Read the model definition and answer for the solid it produces. Units are mm, in the model's axes. A direction names the side the tool comes from. Give positions to 0.01 mm unless a question says otherwise; leave off trailing zeros. Order: outer loops, then holes, each group sorted by start corner. A loop starts at its lowest first (then second) coordinate and runs counter-clockwise, first axis right, second up. Notation, with made-up numbers: (30.5, 88.5) - (79.5, 88.5) arc R25 ccw to (79.5, 105.5) - close; hole circle Ø4 at (28.5, 66). An arc over 180 degrees is marked (long way). Answer as CSV lines item,"result". Start each with the question number.
from build123d import *

# Parameters (mm, degrees)
F0_W     = 6
F0_H     = 6
F0_W_2   = 1
F0_H_2   = 5
F1_DEPTH = 1
F2_DEPTH = 6
F3_R     = 2.49999
F4_R     = 1
F5_DEPTH = 25


# Not quite as in the source:
# - a fillet or chamfer is up to 0.001 mm smaller than in the source, because OpenCascade refuses the exact size


with BuildPart() as f1:
    # F0 (on Top) → F1 (new body)
    with BuildSketch(Plane.XY):
        Rectangle(F0_W, F0_H)
        Polygon((2.5, 2.5), (2.5, -2.5), (1.5, -2.5), (0.5, -2.5), (-0.5, -2.5), (-1.5, -2.5), (-2.5, -2.5), (-2.5, 2.5), (-1.5, 2.5), (-0.5, 2.5), (0.5, 2.5), (1.5, 2.5), align=None, mode=Mode.SUBTRACT)
        with Locations((2, 0)):
            Rectangle(F0_W_2, F0_H_2)
        with Locations((1, 0)):
            Rectangle(F0_W_2, F0_H_2)
        Rectangle(F0_W_2, F0_H_2)
        with Locations((-1, 0)):
            Rectangle(F0_W_2, F0_H_2)
        with Locations((-2, 0)):
            Rectangle(F0_W_2, F0_H_2)
    extrude(amount=F1_DEPTH)

    # F0 (on Top) → F2 (join)
    with BuildSketch(Plane.XY):
        with Locations((1, 0)):
            Rectangle(F0_W_2, F0_H_2)
        with Locations((-1, 0)):
            Rectangle(F0_W_2, F0_H_2)
    extrude(amount=F2_DEPTH)

    # F3 (radius 2.5 in the source; OpenCascade refuses exactly that, so slightly less here)
    f3_edges = [f1.edges().sort_by_distance(p)[0] for p in [
        (-1, -2.5, 6),
        (1, -2.5, 6),
        (-1, 2.5, 6),
        (1, 2.5, 6),
    ]]
    fillet(f3_edges, radius=F3_R)

    # F4 (on face) → F5 (cut)
    with BuildSketch(Plane.YZ.offset(1.5)):
        with Locations((0, 3.5)):
            Circle(F4_R)
    extrude(amount=-F5_DEPTH, mode=Mode.SUBTRACT)


solid = f1.part
(1) Straight lines are drawn through the part: line 1 (Z direction, x = 1.1, y = 0); line 2 (X direction, y = 1.75, z = 2.7); line 3 (Z direction, x = 2.4, y = 1.2). For each, find the intervals that lie inside material, in ascending order. Write a range as [from, to].
(2) Determine the mould class of faces 5 (the cylindrical face through (-0.99, -0.13, 4.49)), 6 (the cylindrical face through (-1, -2, 5)), 7 (the flat face through (0, 0, 0)), 8 (the flat face through (1.5, 0, 2)) for opening direction Z: released by +Z, released by -Z, zero draft, split by the parting line, or undercut.
(3) Section C-C, the plane y = -1.5 is taken. Write down the section's boundary in (x, z), and give its area (3 significant figures).
(4) Section B-B, the plane z = 2.25 is taken. Write down the section's boundary in (x, y).
(5) Flat-ended cylindrical pins translate along their axes: pin 1 Ø2 at (x, y) = (1.5, 2.5) entering from -Z; pin 2 Ø1.5 at (y, z) = (-1, 4.5) entering from +X; pin 3 Ø0.5 at (x, z) = (1, 2.5) entering from -Y; pin 4 Ø0.8 at (x, z) = (-1, 2.5) entering from +Y. Find the tip coordinate at first contact, or state that the pin passes through.
(6) Section A-A, the plane z = 2.9 is taken. Write down the section's boundary in (x, y).
(7) Section D-D, the plane y = 0.4 is taken. Write down the section's boundary in (x, z), and give its area (3 significant figures).
(8) Which of the six approach directions +Z, -Z, +X, -X, +Y, -Y give full straight-line access (tool end or side, diameter ignored) to faces 1 (the flat face through (-1.5, 0, 2)), 2 (the flat face through (1, 2.5, 2)), 3 (the flat face through (0.5, 0, 2)), 4 (the flat face through (-1, -2.5, 2))?
Checks:
1,line 1,"z = [0, 2.5], [4.5, 6]"
1,line 2,"x = [-1.5, -0.5], [0.5, 1.5]"
1,line 3,"z = [0, 1]"
2,face 5,"undercut"
2,face 6,"released by +Z"
2,face 7,"released by -Z"
2,face 8,"zero draft"
3,outline,"(-3, 0) - (3, 0) - (3, 1) - (1.5, 1) - (1.5, 5.5) - (0.5, 5.5) - (0.5, 1) - (-0.5, 1) - (-0.5, 5.5) - (-1.5, 5.5) - (-1.5, 1) - (-3, 1) - close"
3,area,"15.0 mm²"
4,outline,"(-1.5, -2.5) - (-0.5, -2.5) - (-0.5, 2.5) - (-1.5, 2.5) - close; (0.5, -2.5) - (1.5, -2.5) - (1.5, 2.5) - (0.5, 2.5) - close"
5,pin 1,"stops at z = 0"
5,pin 2,"stops at x = 1.5"
5,pin 3,"stops at y = -2.5"
5,pin 4,"stops at y = 2.5"
6,outline,"(-1.5, -2.5) - (-0.5, -2.5) - (-0.5, -0.8) - (-1.5, -0.8) - close; (-1.5, 0.8) - (-0.5, 0.8) - (-0.5, 2.5) - (-1.5, 2.5) - close; (0.5, -2.5) - (1.5, -2.5) - (1.5, -0.8) - (0.5, -0.8) - close; (0.5, 0.8) - (1.5, 0.8) - (1.5, 2.5) - (0.5, 2.5) - close"
7,outline,"(-3, 0) - (3, 0) - (3, 1) - (1.5, 1) - (1.5, 2.58) - (0.5, 2.58) - (0.5, 1) - (-0.5, 1) - (-0.5, 2.58) - (-1.5, 2.58) - (-1.5, 1) - (-3, 1) - close; (-1.5, 4.42) - (-0.5, 4.42) - (-0.5, 5.97) - (-1.5, 5.97) - close; (0.5, 4.42) - (1.5, 4.42) - (1.5, 5.97) - (0.5, 5.97) - close"
7,area,"12.3 mm²"
8,face 1,"+Z, -X, +Y, -Y"
8,face 2,"+Z, +X, -X, +Y"
8,face 3,"+Z, +Y, -Y"
8,face 4,"+Z, +X, -X, -Y"
